Here's how the part is built. I have some questions about the finished solid (model axes, mm). Face numbers are marked on the shaded views. A direction names the side the tool comes from. Give positions to 0.01 mm unless a question says otherwise; leave off trailing zeros. Loops run counter-clockwise (first coordinate to the right, second up) from the corner with the lowest first, then second, coordinate; pieces in that order, holes last.
Q1. If we section it at A-A (z = 0): Please give me the cut outline in (x, y), plus the area to 3 significant figures.
Q2. We'd pull the mould along Z, two halves only. Please class the marked faces 1, 2 and 3: +Z half, -Z half, draft (parallel to the pull), parting line (faces both ways), or undercut.
Q3. For the marked faces 4, 5 and 6, which set-ups out of +Z, -Z, +X, -X, +Y, -Y let a thin tool reach every point of the face, with its end or its side?
Q4. If we section it at C-C (y = 2.85): Please give me the cut outline in (x, z), plus the area to 3 significant figures.
Q5. If we section it at B-B (x = 0): Please give me the cut outline in (y, z), plus the area to 3 significant figures.
Q6. If we section it at D-D (z = 6): Please give me the cut outline in (x, y), plus the area to 3 significant figures.
Q7. I need wall thicknesses on line 1 (X direction, y = 4.25, z = 0); line 2 (X direction, y = 0.85, z = 0); line 3 (Y direction, x = 2.25, z = -7.5). Which ranges of each line are inside material? Lowest first, please.
Q8. Will these pins go through, and if not, where does the flat tip stop? P1, Ø1.6, axis at x = 0, z = 0, coming from the -Y side; P2, Ø1.5, axis at y = 2.5, z = -9, coming from the -X side; P3, Ø2, axis at y = 1.5, z = -7, coming from the +X side; P4, Ø2.5, axis at x = 1, z = -0.5, coming from the +Y side.
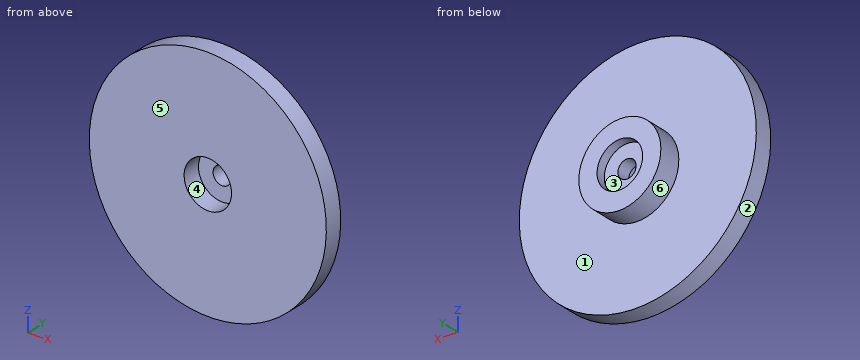
from build123d import *

# Parameters (mm, degrees)
SKETCH_2_R          = 13
EXTRUDE_1_DEPTH     = 2
SKETCH_3_R          = 4.5
SKETCH_3_R_2        = 2.5
EXTRUDE_2_DEPTH     = 2.5
SKETCH_4_R          = 2.5
EXTRUDE_3_DEPTH     = 1.5
SKETCH_5_R          = 2.6
CUT_EXTRUDE_1_DEPTH = 2
SKETCH_6_R          = 1
CUT_EXTRUDE_2_DEPTH = 2


with BuildPart() as part:
    # 草图2 → 凸台-拉伸1 (new body)
    with BuildSketch(Plane(origin=(0, 0, 0), x_dir=(1, 0, 0), z_dir=(0, 1, 0))):
        with Locations(Location((0, 0, 0), (0, 0, 270))):
            Circle(SKETCH_2_R)
    extrude(amount=EXTRUDE_1_DEPTH)

    # 草图3 → 凸台-拉伸2 (add)
    with BuildSketch(Plane(origin=(0, 2, 0), x_dir=(1, 0, 0), z_dir=(0, 1, 0))):
        with Locations(Location((0, 0, 0), (0, 0, 270))):
            Circle(SKETCH_3_R)
        with Locations(Location((0, 0, 0), (0, 0, 270))):
            Circle(SKETCH_3_R_2, mode=Mode.SUBTRACT)
    extrude(amount=EXTRUDE_2_DEPTH)

    # 草图4 → 凸台-拉伸3 (add)
    with BuildSketch(Plane(origin=(0, 2, 0), x_dir=(1, 0, 0), z_dir=(0, 1, 0))):
        with Locations(Location((0, 0, 0), (0, 0, 270))):
            Circle(SKETCH_4_R)
    extrude(amount=EXTRUDE_3_DEPTH)

    # 草图5 → 切除-拉伸1 (cut)
    with BuildSketch(Plane.XZ):
        with Locations(Location((0, 0, 0), (0, 0, 270))):
            Circle(SKETCH_5_R)
    extrude(amount=-CUT_EXTRUDE_1_DEPTH, mode=Mode.SUBTRACT)

    # 草图6 → 切除-拉伸2 (cut)
    with BuildSketch(Plane.XZ.offset(-2)):
        with Locations(Location((0, 0, 0), (0, 0, 270))):
            Circle(SKETCH_6_R)
    extrude(amount=-CUT_EXTRUDE_2_DEPTH, mode=Mode.SUBTRACT)


solid = part.part
Check sheet entries:
1. outline: (-13, 0) - (-2.6, 0) - (-2.6, 2) - (-1, 2) - (-1, 3.5) - (-2.5, 3.5) - (-2.5, 4.5) - (-4.5, 4.5) - (-4.5, 2) - (-13, 2) - close; (1, 2) - (2.6, 2) - (2.6, 0) - (13, 0) - (13, 2) - (4.5, 2) - (4.5, 4.5) - (2.5, 4.5) - (2.5, 3.5) - (1, 3.5) - close
1. area: 56.1 mm2
2. face 1: draft
2. face 2: parting line
2. face 3: undercut
3. face 4: -Y
3. face 5: +Z, -Z, +X, -X, -Y
3. face 6: +Y
4. outline: circle Ø9 at (0, 0); hole circle Ø2 at (0, 0)
4. area: 60.5 mm2
5. outline: (0, -13) - (2, -13) - (2, -4.5) - (4.5, -4.5) - (4.5, -2.5) - (3.5, -2.5) - (3.5, -1) - (2, -1) - (2, -2.6) - (0, -2.6) - close; (0, 2.6) - (2, 2.6) - (2, 1) - (3.5, 1) - (3.5, 2.5) - (4.5, 2.5) - (4.5, 4.5) - (2, 4.5) - (2, 13) - (0, 13) - close
5. area: 56.1 mm2
6. outline: (-11.53, 0) - (11.53, 0) - (11.53, 2) - (-11.53, 2) - close
6. area: 46.1 mm2
7. line 1: x = -4.5 to -2.5, 2.5 to 4.5
7. line 2: x = -13 to -2.6, 2.6 to 13
7. line 3: y = 0 to 2
8. P1: passes through
8. P2: stops at x = -9.89
8. P3: stops at x = 11.53
8. P4: stops at y = 3.5
